Can you work these out from the model? Positions are in its coordinate system, mm. A direction names the side the tool comes from. Give positions to 0.01 mm unless a question says otherwise; leave off trailing zeros. Order: outer loops, then holes, each group sorted by start corner. A loop starts at its lowest first (then second) coordinate and runs counter-clockwise, first axis right, second up. Notation, with made-up numbers: (5, -27) - (61, -27) arc R15 cw to (61, -22) - close; hole circle Ø6 at (-4, 11). An arc over 180 degrees is marked (long way). One line per question, with ' | ' between items.
```python
from build123d import *

# Parameters (mm, degrees)
SURFACE_EXTRUDE1_1_DEPTH = 5
THICKEN1_T2              = 4
BOSS_EXTRUDE1_DEPTH      = 1
FILLET1_R                = 1


with BuildPart() as body_1:
    # Surface-Extrude1: a surface, the sketch's curves swept straight by 5 mm
    with BuildLine(Plane.XY, mode=Mode.PRIVATE) as surface_extrude1_1_path:
        ThreePointArc((17.426406871192846, 25.000000000000007), (-12.573593128807143, 12.573593128807161), (-24.999999999999993, -17.42640687119283))
    surface_extrude1_1 = Shell.extrude(surface_extrude1_1_path.wire(), (0 * SURFACE_EXTRUDE1_1_DEPTH, 0 * SURFACE_EXTRUDE1_1_DEPTH, 1 * SURFACE_EXTRUDE1_1_DEPTH))
    add(Solid.thicken(surface_extrude1_1, -THICKEN1_T2))

    # Sketch2 → Boss-Extrude1 (add)
    with BuildSketch(Plane(origin=(0, 0, 0), x_dir=(-1, 0, 0), z_dir=(0, 0, -1))):
        with BuildLine():
            Line((-17.42640687119285, 29.00000000000001), (-17.426406871192853, 22.000000000000007))
            ThreePointArc((-17.426406871192853, 22.000000000000007), (10.452272785247494, 10.452272785247523), (21.999999999999993, -17.426406871192828))
            Line((21.999999999999993, -17.426406871192828), (24.999999999999993, -17.42640687119283))
            Line((24.999999999999993, -17.42640687119283), (28.999999999999996, -17.426406871192825))
            ThreePointArc((28.999999999999996, -17.426406871192825), (15.402020253553331, 15.402020253553353), (-17.42640687119285, 29.00000000000001))
        make_face()
    extrude(amount=BOSS_EXTRUDE1_DEPTH)

    # Fillet1
    fillet1_edges = [body_1.edges().sort_by_distance(p)[0] for p in [
        (-15.402020253553328, 15.40202025355335, 5),
        (-15.402020253553342, 15.40202025355336, -1),
    ]]
    fillet(fillet1_edges, radius=FILLET1_R)


solid = body_1.part
```
(1) If I drill on line 1 (Z direction, x = 14, y = 23); line 2 (Y direction, x = 11, z = 1.4); line 3 (X direction, y = 9, z = 0.4) (3 decimals), over which ranges is the centre line in solid material (lowest first)?
Answer below:
line 1: -1 to 0 | line 2: 24.51 to 28.55 | line 3: -20.745 to -15.765
(2) Imagine slicing it at A-A (z = 1.45). List the corners of the cut face in (x, y) for me, and give its area (3 significant figures).
Answer below:
outline: (-29, -17.43) - (-25, -17.43) arc R42.43 cw to (17.43, 25) - (17.43, 29) arc R46.43 ccw to start | area: 279 mm^2
(3) Will this pin go through, and if not, where does the flat tip stop? pin 1 (1.5 mm diameter, centred on x = 4.5, z = 0, fed in from +Y).
Answer below:
pin 1: y = 27.37
(4) On a 3-axis mill with a long thin cutter (end or side, diameter ignored), from which of +Z, -Z, +X, -X, +Y, -Y can I reach the whole of each face in a straight line? I mean faces 1 (the face through (-10.1, 10.8, -0.5)), 2 (the face through (-10, 12, 0)). Say none if no direction works.
Answer below:
face 1: +Z, -Z, +X, -Y | face 2: +Z, +X, -Y
